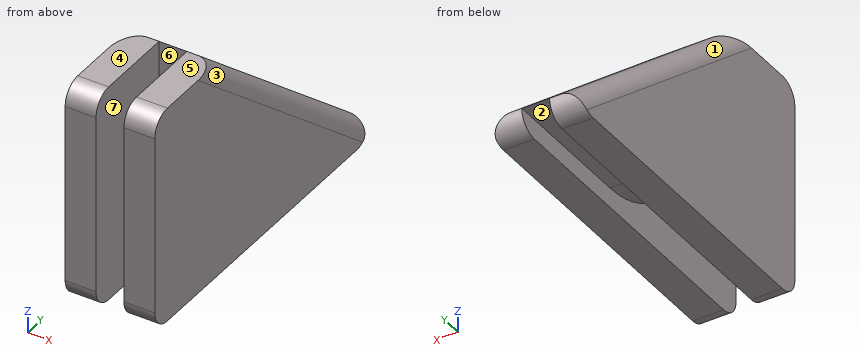
```python
from build123d import *

# Parameters (mm, degrees)
F0_W     = 5
F0_H     = 10
F1_DEPTH = 4.5
F2_W     = 1.4
F2_H     = 5
F3_DEPTH = 25
F4_W     = 1.4
F4_H     = 1
F5_DEPTH = 25
F6_R     = 0.99999
F6_R_2   = 1
F7_R     = 5


# Not quite as in the source:
# - a fillet or chamfer is up to 0.001 mm smaller than in the source, because OpenCascade refuses the exact size


with BuildPart() as f1:
    # F0 (on Right) → F1 (new body)
    with BuildSketch(Plane.YZ):
        with Locations((-2.5, 5)):
            Rectangle(F0_W, F0_H)
        Polygon((0, 10), (0, 0), (12, 0), align=None)
        Polygon((12, 0), (0, 0), (-5, 0), (-5, -1), (12, -1), align=None)
    extrude(amount=F1_DEPTH)

    # F2 (on face) → F3 (cut)
    with BuildSketch(Plane.XY.offset(10)):
        with Locations((2.25, -2.5)):
            Rectangle(F2_W, F2_H)
    extrude(amount=-F3_DEPTH, mode=Mode.SUBTRACT)

    # F4 (on face) → F5 (cut)
    with BuildSketch(Plane(origin=(0, 12, 0), x_dir=(-1, 0, 0), z_dir=(0, 1, 0))):
        with Locations((-2.25, -0.5)):
            Rectangle(F4_W, F4_H)
    extrude(amount=-F5_DEPTH, mode=Mode.SUBTRACT)

    # F6 (call 1 of 8: OpenCascade refuses the feature's edges together) (radius 1 in the source; OpenCascade refuses exactly that, so slightly less here)
    f6_edges = [f1.edges().sort_by_distance(p)[0] for p in [
        (3.725, 12, -1),
    ]]
    fillet(f6_edges, radius=F6_R)

    # F6#2 (call 2 of 8) (radius 1 in the source; OpenCascade refuses exactly that, so slightly less here)
    f6_2_edges = [f1.edges().sort_by_distance(p)[0] for p in [
        (0.775, 12, -1),
    ]]
    fillet(f6_2_edges, radius=F6_R)

    # F6#3 (call 3 of 8)
    f6_3_edges = [f1.edges().sort_by_distance(p)[0] for p in [
        (3.725, -5, -1),
    ]]
    fillet(f6_3_edges, radius=F6_R_2)

    # F6#4 (call 4 of 8)
    f6_4_edges = [f1.edges().sort_by_distance(p)[0] for p in [
        (0.775, -5, -1),
    ]]
    fillet(f6_4_edges, radius=F6_R_2)

    # F6#5 (call 5 of 8)
    f6_5_edges = [f1.edges().sort_by_distance(p)[0] for p in [
        (0.775, -5, 10),
    ]]
    fillet(f6_5_edges, radius=F6_R_2)

    # F6#6 (call 6 of 8)
    f6_6_edges = [f1.edges().sort_by_distance(p)[0] for p in [
        (3.725, -5, 10),
    ]]
    fillet(f6_6_edges, radius=F6_R_2)

    # F6#7 (call 7 of 8)
    f6_7_edges = [f1.edges().sort_by_distance(p)[0] for p in [
        (0, 6, 5),
    ]]
    fillet(f6_7_edges, radius=F6_R_2)

    # F6#8 (call 8 of 8)
    f6_8_edges = [f1.edges().sort_by_distance(p)[0] for p in [
        (4.5, 6, 5),
    ]]
    fillet(f6_8_edges, radius=F6_R_2)

    # F7
    f7_edges = [f1.edges().sort_by_distance(p)[0] for p in [
        (2.25, 0, 0),
    ]]
    fillet(f7_edges, radius=F7_R)


solid = f1.part
```
The model under review builds one solid part; all positions refer to its coordinate system, in mm. Face numbers are marked on the shaded views. A direction names the side the tool comes from. Round coordinates to 2 decimals unless told otherwise and drop trailing zeros. Loops run counter-clockwise (first coordinate to the right, second up) from the corner with the lowest first, then second, coordinate; pieces in that order, holes last.
1) Wall thickness on line 1 along X through (y, z) = (0.5, 0.25); line 2 along Z through (x, y) = (1.45, 2.25) (3 decimals); line 3 along Y through (x, z) = (2.5, 1.5): over which ranges is each line inside the solid? List them lowest first.
Values follow:
line 1: x = 0 to 1.55, 2.95 to 4.5
line 2: z = -1 to 8.125
line 3: y = 1.43 to 10.2
2) Consider section D-D on x = 0.65. State the section outline as (y, z) points.
Values follow:
outline: (-5, 0) arc R1 ccw to (-4, -1) - (11, -1) arc R1 ccw to (12, -0.08) - (-0.1, 10) - (-4, 10) arc R1 ccw to (-5, 9) - close
3) The part is to be moulded in two halves that separate along X. For the marked faces 1, 2, 3 and 4, say which applies: pulls with the +X half, pulls with the -X half, needs draft (parallel to the pull), parting line crosses it, or undercut.
Values follow:
face 1: pulls with the -X half
face 2: undercut
face 3: pulls with the +X half
face 4: needs draft
4) Tool access review of the marked faces 5, 6 and 7: name each direction out of +Z, -Z, +X, -X, +Y, -Y from which nothing blocks a thin tool from reaching the whole face with its end or side.
Values follow:
face 5: +Z, +X, -X, +Y, -Y
face 6: +Z, -Z, -Y
face 7: -Z, -Y
5) Consider section A-A on y = -3. State the section outline as (x, z) points.
Values follow:
outline: (0, -1) - (1.55, -1) - (1.55, 10) - (0, 10) - close; (2.95, -1) - (4.5, -1) - (4.5, 10) - (2.95, 10) - close
6) Consider section C-C on x = 1.95. State the section outline as (y, z) points.
Values follow:
outline: (0, 5) arc R5 ccw to (5, 0) - (12, 0) - (0, 10) - close
